Read the model definition and answer for the solid it produces. Units are mm, in the model's axes. Face numbers are marked on the shaded views. A direction names the side the tool comes from. Round coordinates to 2 decimals unless told otherwise and drop trailing zeros. Order: outer loops, then holes, each group sorted by start corner. A loop starts at its lowest first (then second) coordinate and runs counter-clockwise, first axis right, second up.
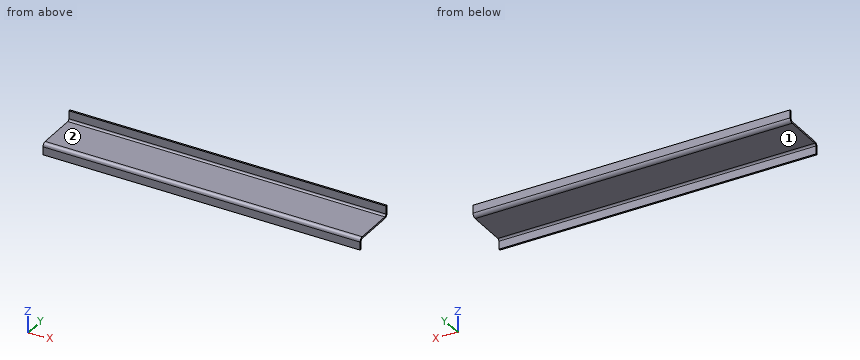
from build123d import *

# Parameters (mm, degrees)
SKETCH1_W                    = 273
SKETCH1_H                    = 39.5
BASE_FLANGE1_DEPTH           = 1.5
EDGE_FLANGE1_STRIP_W         = 9.2
EDGE_FLANGE1_STRIP_H         = 1.5
EDGE_FLANGE1_STRIP_CUT_DEPTH = 273
EDGE_FLANGE1_DEPTH           = 273
EDGE_FLANGE2_STRIP_W         = 9.2
EDGE_FLANGE2_STRIP_H         = 1.5
EDGE_FLANGE2_STRIP_CUT_DEPTH = 273
EDGE_FLANGE2_DEPTH           = 273


# Sheet-metal steps are written as plain solids
with BuildPart() as part:
    # Sketch1 → Base-Flange1 (new body)
    with BuildSketch(Plane.XY):
        Rectangle(SKETCH1_W, SKETCH1_H)
    extrude(amount=-BASE_FLANGE1_DEPTH)

    # Edge-Flange1 strip (across the edge) → Edge-Flange1 strip cut (cut)
    with BuildSketch(Plane(origin=(136.5, 19.75, 0), x_dir=(0, -1, 0), z_dir=(-1, 0, 0))):
        with Locations((-1.5, -0.75)):
            Rectangle(EDGE_FLANGE1_STRIP_W, EDGE_FLANGE1_STRIP_H)
    extrude(amount=EDGE_FLANGE1_STRIP_CUT_DEPTH, mode=Mode.SUBTRACT)

    # Edge-Flange1 section (across the edge) → Edge-Flange1 (add)
    with BuildSketch(Plane(origin=(136.5, 19.75, 0), x_dir=(0, -1, 0), z_dir=(-1, 0, 0))):
        with BuildLine():
            Line((0, 1.6), (0, 8.5))
            Line((0, 8.5), (1.5, 8.5))
            Line((1.5, 8.5), (1.5, 1.6))
            ThreePointArc((1.5, 1.6), (1.96862915, 0.46862915), (3.1, 0))
            Line((3.1, 0), (3.1, -1.5))
            ThreePointArc((3.1, -1.5), (0.907968978, -0.592031022), (0, 1.6))
        make_face()
    extrude(amount=EDGE_FLANGE1_DEPTH)

    # Edge-Flange2 strip (across the edge) → Edge-Flange2 strip cut (cut)
    with BuildSketch(Plane(origin=(136.5, -19.75, -1.5), x_dir=(0, 1, 0), z_dir=(-1, 0, 0))):
        with Locations((-1.5, -0.75)):
            Rectangle(EDGE_FLANGE2_STRIP_W, EDGE_FLANGE2_STRIP_H)
    extrude(amount=EDGE_FLANGE2_STRIP_CUT_DEPTH, mode=Mode.SUBTRACT)

    # Edge-Flange2 section (across the edge) → Edge-Flange2 (add)
    with BuildSketch(Plane(origin=(136.5, -19.75, -1.5), x_dir=(0, 1, 0), z_dir=(-1, 0, 0))):
        with BuildLine():
            Line((0, 1.6), (0, 8.5))
            Line((0, 8.5), (1.5, 8.5))
            Line((1.5, 8.5), (1.5, 1.6))
            ThreePointArc((1.5, 1.6), (1.96862915, 0.46862915), (3.1, 0))
            Line((3.1, 0), (3.1, -1.5))
            ThreePointArc((3.1, -1.5), (0.907968978, -0.592031022), (0, 1.6))
        make_face()
    extrude(amount=EDGE_FLANGE2_DEPTH)


solid = part.part
Q1. Straight lines are drawn through the part: probe 1 along Z at (x, y) = (124, 10.5); probe 2 along Y at (x, z) = (-5, 6); probe 3 along Y at (x, z) = (-93, -7.25). For each, find the intervals that lie inside material, in ascending order.
Outcome:
probe 1: z = -1.5 to 0
probe 2: y = 18.25 to 19.75
probe 3: y = -19.75 to -18.25
Q2. For the marked faces 1 and 2, determine the directions among +Z, -Z, +X, -X, +Y, -Y from which every point of the face is accessible in a straight line to the end or side of a thin tool.
Outcome:
face 1: -Z, +X, -X, +Y
face 2: +Z, +X, -X, -Y
Q3. A cutting plane is placed at A-A, the plane x = 117.5. Give the vertices of the cut face in (y, z).
Outcome:
outline: (-19.75, -10) - (-18.25, -10) - (-18.25, -3.1) arc R1.6 cw to (-16.65, -1.5) - (16.65, -1.5) arc R3.1 ccw to (19.75, 1.6) - (19.75, 8.5) - (18.25, 8.5) - (18.25, 1.6) arc R1.6 cw to (16.65, 0) - (-16.65, 0) arc R3.1 ccw to (-19.75, -3.1) - close
Q4. A cutting plane is placed at C-C, the plane y = -5. Give the vertices of the cut face in (x, z).
Outcome:
outline: (-136.5, -1.5) - (136.5, -1.5) - (136.5, 0) - (-136.5, 0) - close
Q5. A cutting plane is placed at B-B, the plane z = -7.75. Give the vertices of the cut face in (x, y).
Outcome:
outline: (-136.5, -19.75) - (136.5, -19.75) - (136.5, -18.25) - (-136.5, -18.25) - close
Q6. Flat-ended cylindrical pins translate along their axes: pin 1 (16.5 mm diameter, centred on x = 20.5, y = 5, fed in from +Z); pin 2 (8 mm diameter, centred on y = -3.5, z = 3, fed in from -X); pin 3 (3.5 mm diameter, centred on x = -51.5, z = -7, fed in from +Y); pin 4 (8 mm diameter, centred on x = 90, y = 1, fed in from -Z). Find the tip coordinate at first contact, or state that the pin passes through.
Outcome:
pin 1: stops at z = 0
pin 2: stops at x = -136.5
pin 3: stops at y = -18.25
pin 4: stops at z = -1.5
